Read the model definition and answer for the solid it produces. Units are mm, in the model's axes. A direction names the side the tool comes from. Round coordinates to 2 decimals unless told otherwise and drop trailing zeros. Order: outer loops, then holes, each group sorted by start corner. A loop starts at its lowest first (then second) coordinate and runs counter-clockwise, first axis right, second up. Notation, with made-up numbers: (-7, 40) - (29, 40) arc R20 cw to (29, 60) - close; hole circle Ø1 at (85.5, -4). An arc over 180 degrees is marked (long way). Answer as a JSON object with one key per item and string values. Group by question number.
Q1. A cutting plane is placed at B-B on y = -23. Determine the outline of the cut face in (x, z).
Q2. Consider line 1 (Y direction, x = 0, z = 13.85); line 2 (Z direction, x = 0, y = -23); line 3 (Z direction, x = 0, y = -10). Determine where each line is inside the solid, lowest interval first.
Q3. A cutting plane is placed at D-D on y = -5. Determine the outline of the cut face in (x, z).
Q4. Given pin 1 Ø2.5 at (x, y) = (-2, -2) entering from -Z; pin 2 Ø2 at (y, z) = (-5, -2.5) entering from -X; pin 3 Ø2 at (y, z) = (-18, -5.5) entering from -X, each flat-ended and moving along its own axis, determine where each tip first touches the part or whether it passes through.
Q5. The mould has two halves that part along Z. Classify faces 1 (the flat face through (0, -12, 15)), 2 (the flat face through (0, -21, 9)), 3 (the flat face through (-4, -21, 10)), 4 (the cylindrical face through (0, -18, 14)): pulls with the +Z half, pulls with the -Z half, needs draft (parallel to the pull), parting line crosses it, or undercut.
Q6. A tool of negligible diameter and unlimited length cuts with its end or side. For faces 5 (the flat face through (4, -21, 10)), 6 (the flat face through (0, -4, 9)), 7 (the flat face through (10.5, -12, 7)), from which of +Z, -Z, +X, -X, +Y, -Y can it reach the whole face along a straight path? Write none if from no direction.
Q7. A cutting plane is placed at A-A on x = 0. Determine the outline of the cut face in (y, z).
Q8. A cutting plane is placed at C-C on z = -2.75. Determine the outline of the cut face in (x, y), and give its area (3 significant figures).
```python
from build123d import *

# Parameters (mm, degrees)
F1_DEPTH        = 25
F2_R            = 2
F3_DEPTH        = 6
F4_W            = 8
F4_H            = 3
F5_DEPTH        = 8
F5_COPIES_COUNT = 2
F5_COPIES_PITCH = 17


# Not quite as in the source:
# - a pattern or mirror of a feature is missing from the dataset's text; its kind, count and spacing are read off the source's solid


with BuildPart() as f1:
    # F0 (on Front) → F1 (new body)
    with BuildSketch(Plane.XZ):
        with BuildLine():
            ThreePointArc((-10.5, 0), (0, 10.5), (10.5, 0))
            Line((10.5, 0), (10.5, 15))
            Line((10.5, 15), (-10.5, 15))
            Line((-10.5, 15), (-10.5, 0))
        make_face()
        with BuildLine():
            Line((10.5, 0), (7.5, 0))
            ThreePointArc((7.5, 0), (0, -7.5), (-7.5, 0))
            Line((-7.5, 0), (-10.5, 0))
            ThreePointArc((-10.5, 0), (0, -10.5), (10.5, 0))
        make_face()
        with BuildLine():
            ThreePointArc((-7.5, 0), (0, 7.5), (7.5, 0))
            Line((7.5, 0), (10.5, 0))
            ThreePointArc((10.5, 0), (0, 10.5), (-10.5, 0))
            Line((-10.5, 0), (-7.5, 0))
        make_face()
    extrude(amount=F1_DEPTH)

    # F2 (on face) → F3 (cut)
    with BuildSketch(Plane.XY.offset(15)):
        with Locations((0, -5)):
            Circle(F2_R)
        with Locations((0, -20)):
            Circle(F2_R)
    extrude(amount=-F3_DEPTH, mode=Mode.SUBTRACT)

    # F4 (on face) → F5 (cut)
    with BuildSketch(Plane.XZ.offset(25)):
        with Locations((0, 10.5)):
            Rectangle(F4_W, F4_H)
    f5 = extrude(amount=-F5_DEPTH, mode=Mode.SUBTRACT)

    # F5_copies: F5 ×2
    with Locations(*[(0, i * F5_COPIES_PITCH, 0) for i in range(1, F5_COPIES_COUNT)]):
        add(f5, mode=Mode.SUBTRACT)


solid = f1.part
```
Result set:
{
 "1": {"outline": "(-10.5, 0) arc R10.5 ccw to (10.5, 0) - (10.5, 15) - (-10.5, 15) - close; hole circle Ø15 at (0, 0); hole (-4, 9) - (4, 9) - (4, 12) - (-4, 12) - close"},
 "2": {"line 1": "y = -25 to -22, -18 to -7, -3 to 0", "line 2": "z = -10.5 to -7.5, 7.5 to 9, 12 to 15", "line 3": "z = -10.5 to -7.5, 7.5 to 15"},
 "3": {"outline": "(-10.5, 0) arc R10.5 ccw to (10.5, 0) - (10.5, 15) - (2, 15) - (2, 12) - (4, 12) - (4, 9) - (-4, 9) - (-4, 12) - (-2, 12) - (-2, 15) - (-10.5, 15) - close; hole circle Ø15 at (0, 0)"},
 "4": {"pin 1": "stops at z = -10.47", "pin 2": "stops at x = -10.39", "pin 3": "stops at x = -9.49"},
 "5": {"face 1": "pulls with the +Z half", "face 2": "undercut", "face 3": "undercut", "face 4": "needs draft"},
 "6": {"face 5": "-Y", "face 6": "+Y", "face 7": "+Z, -Z, +X, +Y, -Y"},
 "7": {"outline": "(-25, -10.5) - (0, -10.5) - (0, -7.5) - (-25, -7.5) - close; (-25, 7.5) - (0, 7.5) - (0, 9) - (-8, 9) - (-8, 12) - (-7, 12) - (-7, 15) - (-18, 15) - (-18, 12) - (-17, 12) - (-17, 9) - (-25, 9) - close; (-25, 12) - (-22, 12) - (-22, 15) - (-25, 15) - close; (-3, 12) - (0, 12) - (0, 15) - (-3, 15) - close"},
 "8": {"outline": "(-10.13, -25) - (-6.98, -25) - (-6.98, 0) - (-10.13, 0) - close; (6.98, -25) - (10.13, -25) - (10.13, 0) - (6.98, 0) - close", "area": "158 mm²"}
}
